Build history of the part. All positions in model axes, mm. Coordinates: 2 decimals unless noted, no trailing zeros. Order: outer loops, then holes, each group sorted by start corner. A loop starts at its lowest first (then second) coordinate and runs counter-clockwise, first axis right, second up. Notation, with made-up numbers: (44, -19) - (75, -19) arc R7 ccw to (75, -7) - close; hole circle Ø9 at (25.25, 26.25). An arc over 180 degrees is marked (long way). One line per item, written item: value.
from build123d import *

# Parameters (mm, degrees)
SKETCH_1_R          = 2
EXTRUDE_1_DEPTH     = 1.5
HOLE_WIZARD_3_D     = 3.15
HOLE_WIZARD_3_DEPTH = 12
HOLE_WIZARD_3_TIP   = 0.946355475


with BuildPart() as part:
    # Эскиз1 → Бобышка-Вытянуть1 (new body)
    with BuildSketch(Plane(origin=(0, 0, 0), x_dir=(1, 0, 0), z_dir=(0, 1, 0))):
        with BuildLine():
            Line((0, 0), (80, 0))
            Line((80, 0), (80, 20))
            Line((80, 20), (62.470537173, 20))
            ThreePointArc((62.470537173, 20), (54, 16.5), (45.529462827, 20))
            Line((45.529462827, 20), (0, 20))
            Line((0, 20), (0, 0))
        make_face()
        with Locations((15, 10.5)):
            Circle(SKETCH_1_R, mode=Mode.SUBTRACT)
    extrude(amount=EXTRUDE_1_DEPTH)

    # Под_М3
    with Locations(Plane.XZ):
        with Locations((75, -6), (3, -17)):
            Hole(HOLE_WIZARD_3_D / 2, depth=HOLE_WIZARD_3_DEPTH)
            with Locations((0, 0, -(HOLE_WIZARD_3_DEPTH + HOLE_WIZARD_3_TIP / 2))):  # 118° drill point
                Cone(0, HOLE_WIZARD_3_D / 2, HOLE_WIZARD_3_TIP, mode=Mode.SUBTRACT)


solid = part.part
1. Band-saw the part on C-C, the plane x = 75. Give the cut face in (y, z) (3 decimals), and give its area (3 significant figures).
Values found:
outline: (0, -20) - (1.5, -20) - (1.5, -7.575) - (0, -7.575) - close; (0, -4.425) - (1.5, -4.425) - (1.5, 0) - (0, 0) - close
area: 25.3 mm2
2. Flat gauge pin, fed straight in: P1, Ø1.9, axis at x = 3, z = -17, coming from the +Y side. Where does the tip first touch, or does it go through?
Values found:
P1: passes through
3. Band-saw the part on A-A, the plane y = 1.25. Give the cut face in (x, z) (3 decimals), and give its area (3 significant figures).
Values found:
outline: (0, -20) - (45.529, -20) arc R12 cw to (62.471, -20) - (80, -20) - (80, 0) - (0, 0) - close; hole circle Ø3.15 at (3, -17); hole circle Ø4 at (15, -10.5); hole circle Ø3.15 at (75, -6)
area: 1,530 mm2
4. Band-saw the part on B-B, the plane z = -6. Give the cut face in (x, y) (3 decimals), and give its area (3 significant figures).
Values found:
outline: (0, 0) - (73.425, 0) - (73.425, 1.5) - (0, 1.5) - close; (76.575, 0) - (80, 0) - (80, 1.5) - (76.575, 1.5) - close
area: 115 mm2
5. Band-saw the part on D-D, the plane x = 61.5. Give the cut face in (y, z), and give its area (3 significant figures).
Values found:
outline: (0, -19.13) - (1.5, -19.13) - (1.5, 0) - (0, 0) - close
area: 28.7 mm2
6. Two-plate mould, pull along Z, no slides. Class faces 1 (the face through (71, 1, -20)), 2 (the face through (2.273, 0.761, -18.397)), 3 (the face through (39, 1, 0)): pulls with the +Z half, pulls with the -Z half, needs draft (parallel to the pull), parting line crosses it, or undercut.
Values found:
face 1: pulls with the -Z half
face 2: undercut
face 3: pulls with the +Z half
7. Probe line 1 along Z through (x, y) = (15, 1); line 2 along Z through (x, y) = (3, 0.65) (3 decimals); line 3 along X through (y, z) = (0.6, -10.5). List the from-to ranges inside material, lowest first.
Values found:
line 1: z = -20 to -12.5, -8.5 to 0
line 2: z = -20 to -18.575, -15.425 to 0
line 3: x = 0 to 13, 17 to 80
